Read the model definition and answer for the solid it produces. Units are mm, in the model's axes. Give positions to 0.01 mm unless a question says otherwise; leave off trailing zeros. Write each loop counter-clockwise with the first axis right and the second up, starting at its lowest first coordinate (ties: lowest second). Pieces come first, ordered by that corner, then holes. Notation, with made-up numbers: (23.5, 9.25) -> (67.5, 9.25) arc R37 ccw to (67.5, 46.25) -> close; hole circle Ø7 at (59.5, 61.25). An arc over 180 degrees is marked (long way). Write item = value, one per line.
from build123d import *

# Parameters (mm, degrees)
F0_W     = 150
F0_H     = 120
F1_DEPTH = 280
F3_DEPTH = 150


with BuildPart() as f1:
    # F0 (on Top) → F1 (new body)
    with BuildSketch(Plane.XY):
        with Locations((-1.511779, 0.179398)):
            Rectangle(F0_W, F0_H)
    extrude(amount=F1_DEPTH)

    # F2 (on face) → F3 (cut, through all)
    with BuildSketch(Plane(origin=(-76.511779, 0, 0), x_dir=(0, -1, 0), z_dir=(-1, 0, 0))):
        Polygon((-60.179398, 262.2087), (0, 280), (-60.179398, 280), align=None)
        Polygon((59.820602, 280), (0, 280), (59.820602, 261.037251), align=None)
    extrude(amount=-F3_DEPTH, mode=Mode.SUBTRACT)


solid = f1.part
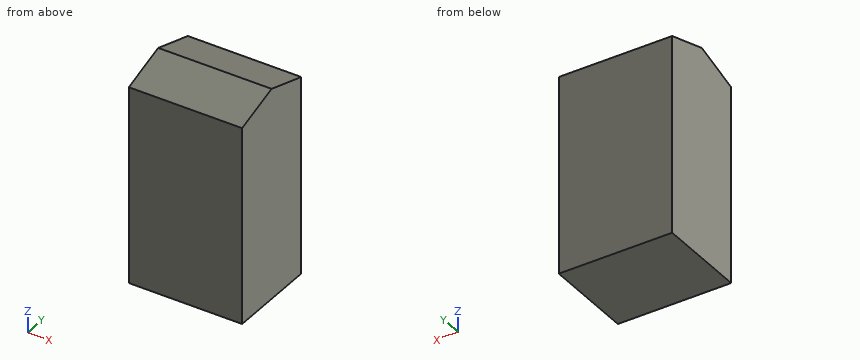
(1) The part is cut by section A-A on x = 19.5. Determine the outline of the cut face in (y, z).
Checks:
outline = (-59.82, 0) -> (60.18, 0) -> (60.18, 262.21) -> (0, 280) -> (-59.82, 261.04) -> close
(2) The part is cut by section C-C on y = 21.5. Determine the outline of the cut face in (x, z).
Checks:
outline = (-76.51, 0) -> (73.49, 0) -> (73.49, 273.64) -> (-76.51, 273.64) -> close
(3) The part is cut by section B-B on y = 43.5. Determine the outline of the cut face in (x, z).
Checks:
outline = (-76.51, 0) -> (73.49, 0) -> (73.49, 267.14) -> (-76.51, 267.14) -> close
(4) Given P1, Ø8, axis at x = 8.5, y = 16, coming from the +Z side; P2, Ø3, axis at x = -52, y = -42, coming from the +Z side, each flat-ended and moving along its own axis, determine where each tip first touches the part or whether it passes through.
Checks:
P1 = 276.45
P2 = 267.16
(5) Consider L1, parallel to Z at x = 12.5, y = 25; L2, parallel to Z at x = 29.5, y = 44.5. Determine where each line is inside the solid, lowest interval first.
Checks:
L1 = 0 to 272.61
L2 = 0 to 266.84
